Autodesk Inventor part; units mm, degrees
ref_plane "YZ Plane" through (0, 0, 0) normal (1, 0, 0) x (0, 1, 0)
ref_plane "XZ Plane" through (0, 0, 0) normal (0, 1, 0) x (-1, 0, 0)
ref_plane "XY Plane" through (0, 0, 0) normal (0, 0, 1) x (1, 0, 0)
sketch "Sketch1" plane through (0, 0, 0) normal (0, 1, 0) x (-1, 0, 0)
  line L0 (3.8, 11.75) -> (-3.8, 11.75)
  line L1 (-3.8, 11.75) -> (-3.8, -11.75)
  line L2 (-3.8, -11.75) -> (3.8, -11.75)
  line L3 (3.8, -11.75) -> (3.8, 11.75)
  circle A0 centre (0, 9.1) radius 1.6
  circle A1 centre (0, -9.1) radius 1.6
  point P0 (0, 0)
  dimension "d0" = 23.5
  dimension "d1" = 7.6
  dimension "d2" = 11.75
  dimension "d3" = 3.8
  dimension "d4" = 3.2
  dimension "d5" = 3.2
  dimension "d6" = 18.2
  dimension "d7" = 9.1
extrude "Extrusion1" add sketch "Sketch1" along normal blind 2.4
fillet "Fillet1" radius 1 4 edges at (3.8, 1.2, 11.75) (-3.8, 1.2, 11.75) (3.8, 1.2, -11.75) (-3.8, 1.2, -11.75)
sketch "Sketch2" plane through (0, 2.4, 0) normal (0, 1, 0) x (1, 0, 0)
  line L0 (-3.05, -4.6194) -> (-3.05, 4.6194)
  line L1 (-3.05, 4.6194) -> (3.05, 6.85)
  line L2 (3.05, 6.85) -> (3.05, -6.85)
  line L3 (3.05, -6.85) -> (-3.05, -4.6194)
  line L4 (2.55, -6.1348) -> (-2.55, -4.2698)
  line L5 (-2.55, -4.2698) -> (-2.55, 4.2698)
  line L6 (-2.55, 4.2698) -> (2.55, 6.1348)
  line L7 (2.55, 6.1348) -> (2.55, -6.1348)
  point P0 (0, 0)
  dimension "d11" = 69.914
  dimension "d13" = 13.7
  dimension "d14" = 6.1
  dimension "d15" = 3.05
  dimension "d17" = 0.5
  dimension "d18" = 0.5
  dimension "d19" = 0.5
  dimension "d20" = 0.5
  dimension "d21" = 6.85
  dimension "d22" = 69.914
  dimension "d23" = 69.914
extrude "Extrusion2" add sketch "Sketch2" along normal blind 4.6
fillet "Fillet2" radius 1 8 edges at (-3.05, 4.7, -4.6194) (-3.05, 4.7, 4.6194) (3.05, 4.7, 6.85) (3.05, 4.7, -6.85) (-2.55, 4.7, -4.2698) (-2.55, 4.7, 4.2698) (2.55, 4.7, -6.1348) (2.55, 4.7, 6.1348)
sketch "Sketch3" plane through (0, 0, 0) normal (0, -1, 0) x (1, 0, 0)
  line L0 (3.4, 6.9) -> (-3.4, 6.9)
  line L1 (-3.4, 6.9) -> (-3.4, -6.9)
  line L2 (-3.4, -6.9) -> (3.4, -6.9)
  line L3 (3.4, -6.9) -> (3.4, 6.9)
  point P0 (0, 0)
  dimension "d27" = 13.8
  dimension "d28" = 6.8
  dimension "d29" = 6.9
  dimension "d30" = 3.4
extrude "Extrusion3" add sketch "Sketch3" along normal blind 3.5
equation "\"d5\" = d4"
equation "\"d22\" = d11"
properties part number "15pin female connector"
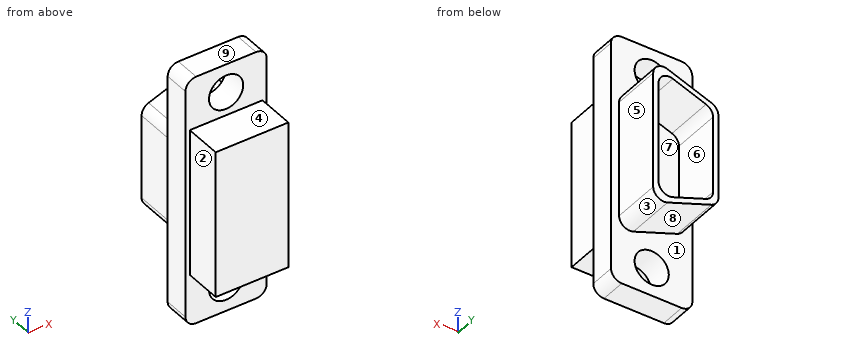
The listing builds one solid part. Answer for the finished solid, in the listing's coordinates (mm). Face numbers are marked on the shaded views. A direction names the side the tool comes from. Round coordinates to 2 decimals unless told otherwise and drop trailing zeros. Loops run counter-clockwise (first coordinate to the right, second up) from the corner with the lowest first, then second, coordinate; pieces in that order, holes last. Notation, with made-up numbers: M 12,80.25 L 34,80.25 A15 cw 34,93.25 Z; hole C 80.25,24 d9. An arc over 180 degrees is marked long. Write each question's results on one line, items separated by ' | '. Start each with the question number.
1) Find section D-D on z = 1.25. Write down the section's boundary in (x, y), plus the area to 3 significant figures.
2) Find section A-A on z = -9.1. Write down the section's boundary in (x, y).
3) Which of the six approach directions +Z, -Z, +X, -X, +Y, -Y give full straight-line access (tool end or side, diameter ignored) to the marked faces 1, 2, 3, 4 and 5?
4) Determine the mould class of the marked faces 6, 7, 8 and 9 for opening direction X: pulls with the +X half, pulls with the -X half, needs draft (parallel to the pull), parting line crosses it, or undercut.
5) Straight lines are drawn through the part: probe 1 along Z at (x, y) = (-0.75, 1); probe 2 along Z at (x, y) = (-0.5, 0.75); probe 3 along Y at (x, z) = (1.5, 8). For each, find the intervals that lie inside material, in ascending order.
6) Find section C-C on x = 0. Write down the section's boundary in (y, z).
7) Each of these flat-tipped pins is pushed along its axis until it touches: pin 1 (3 mm diameter, centred on x = 1, z = 0.5, fed in from +Y); pin 2 (2.5 mm diameter, centred on x = -1.5, z = -6, fed in from +Y); pin 3 (5 mm diameter, centred on y = 5, z = -1.5, fed in from +X); pin 4 (2.5 mm diameter, centred on y = 4, z = 1, fed in from -X). Where does it stop, or does it pass through?
8) Find section B-B on y = 0.75. Write down the section's boundary in (x, z).
Final values:
1) outline: M -3.8,0 L -3.4,0 L -3.4,-3.5 L 3.4,-3.5 L 3.4,0 L 3.8,0 L 3.8,2.4 L 3.05,2.4 L 3.05,7 L 2.55,7 L 2.55,2.4 L -2.55,2.4 L -2.55,7 L -3.05,7 L -3.05,2.4 L -3.8,2.4 Z | area: 46.6 mm²
2) outline: M -3.8,0 L -1.6,0 L -1.6,2.4 L -3.8,2.4 Z; M 1.6,0 L 3.8,0 L 3.8,2.4 L 1.6,2.4 Z
3) face 1: +Y | face 2: +Z, -Z, -X, -Y | face 3: -Z, +Y | face 4: +Z, +X, -X, -Y | face 5: +Z, -Z, +X, +Y
4) face 6: undercut | face 7: undercut | face 8: pulls with the -X half | face 9: needs draft
5) probe 1: -11.75 to -10.51, -7.69 to 7.69, 10.51 to 11.75 | probe 2: -11.75 to -10.62, -7.58 to 7.58, 10.62 to 11.75 | probe 3: 0 to 2.4
6) outline: M -3.5,-6.9 L 0,-6.9 L 0,-7.5 L 2.4,-7.5 L 2.4,-5.73 L 7,-5.73 L 7,-5.2 L 2.4,-5.2 L 2.4,5.2 L 7,5.2 L 7,5.73 L 2.4,5.73 L 2.4,7.5 L 0,7.5 L 0,6.9 L -3.5,6.9 Z; M 0,-11.75 L 2.4,-11.75 L 2.4,-10.7 L 0,-10.7 Z; M 0,10.7 L 2.4,10.7 L 2.4,11.75 L 0,11.75 Z
7) pin 1: y = 2.4 | pin 2: y = 7 | pin 3: x = 3.05 | pin 4: x = -3.05
8) outline: M -3.8,-10.75 A1 ccw -2.8,-11.75 L 2.8,-11.75 A1 ccw 3.8,-10.75 L 3.8,10.75 A1 ccw 2.8,11.75 L -2.8,11.75 A1 ccw -3.8,10.75 Z; hole C 0,-9.1 d3.2; hole C 0,9.1 d3.2
